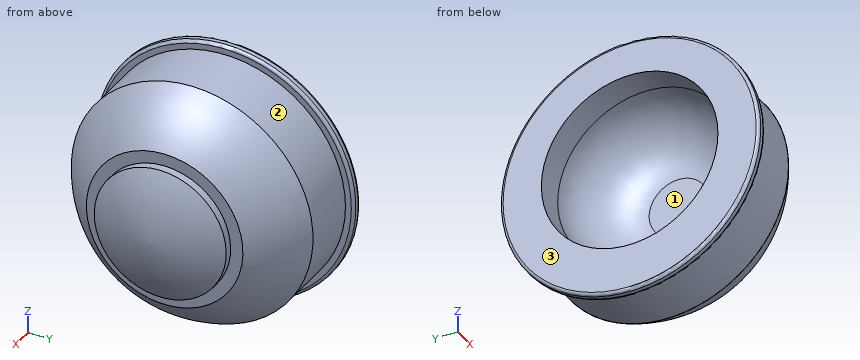
```python
from build123d import *

# Parameters (mm, degrees)
F0_R     = 20.5
F1_DEPTH = 10
F4_R     = 22
F5_DEPTH = 1.7
F6_R     = 0.5
F7_R     = 15
F8_DEPTH = 15
F9_R     = 10


with BuildPart() as f1:
    # F0 (on Right) → F1 (new body)
    with BuildSketch(Plane.YZ):
        Circle(F0_R)
    extrude(amount=F1_DEPTH)

    # F2 (on Front) → F3 (revolve)
    with BuildSketch(Plane.XZ):
        with BuildLine():
            Line((10, 0), (23.039928, 0))
            ThreePointArc((23.039928, 0), (22.111209, 5.803276), (19.804215, 11.208673))
            Line((19.804215, 11.208673), (18.443597, 11.208673))
            Line((18.443597, 11.208673), (18.443597, 13.296706))
            ThreePointArc((18.443597, 13.296706), (14.6452, 17.40848), (10, 20.532038))
            Line((10, 20.532038), (10, 0))
        make_face()
    revolve(axis=Axis((11.340726, 0, 0), (1, 0, 0)))

    # F4 (on face) → F5 (join)
    with BuildSketch(Plane(origin=(0, 0, 0), x_dir=(0, -1, 0), z_dir=(-1, 0, 0))):
        Circle(F4_R)
    extrude(amount=F5_DEPTH)

    # F6
    f6_edges = [f1.edges().sort_by_distance(p)[0] for p in [
        (-1.7, 22, 0),
        (0, 22, 0),
    ]]
    fillet(f6_edges, radius=F6_R)

    # F7 (on face) → F8 (cut)
    with BuildSketch(Plane(origin=(-1.7, 0, 0), x_dir=(0, -1, 0), z_dir=(-1, 0, 0))):
        with Locations((0, 0.914327)):
            Circle(F7_R)
    extrude(amount=-F8_DEPTH, mode=Mode.SUBTRACT)

    # F9
    f9_edges = [f1.edges().sort_by_distance(p)[0] for p in [
        (13.3, 15, 0.914327),
    ]]
    fillet(f9_edges, radius=F9_R)


solid = f1.part
```
Can you work these out from the model? Positions are in its coordinate system, mm. Face numbers are marked on the shaded views. Give positions to 0.01 mm unless a question says otherwise; leave off trailing zeros. Use CSV: the item, a comma, the result in double quotes. Start each with the question number.
1. For P1, Ø5, axis at y = 14, z = -3, coming from the -X side; P2, Ø5, axis at x = 11, z = 14.5, coming from the -Y side; P3, Ø1, axis at x = 20, y = 8.5, coming from the +Z side; P4, Ø8, axis at x = 9, y = -10.5, coming from the -Z side, each with a flat end and sliding along its axis, tell me the tip position at first contact or that it passes through.
2. If we mould it in two halves opening along Z, with no side actions, what happens to the marked faces 1, 2 and 3? For each: released by +Z, released by -Z, zero draft, split by the parting line, or undercut.
3. If I drill on L1, parallel to Z at x = -0.6, y = 0; L2, parallel to Z at x = 1.7, y = 0; L3, parallel to Y at x = 4.25, z = -2.5, over which ranges is the centre line in solid material (lowest first)?
Response values:
1,P1,"x = -1.7"
1,P2,"y = -16.51"
1,P3,"z = 7.81"
1,P4,"z = -19.44"
2,face 1,"undercut"
2,face 2,"split by the parting line"
2,face 3,"zero draft"
3,L1,"-22 to -14.09, 15.91 to 22"
3,L2,"-20.5 to -14.09, 15.91 to 20.5"
3,L3,"-20.35 to -14.56, 14.56 to 20.35"
